from build123d import *

# Parameters (mm, degrees)
SKETCH1_R               = 8
BOSS_EXTRUDE1_DEPTH     = 26.25
SKETCH2_R               = 6
BOSS_EXTRUDE2_DEPTH     = 21.875
SKETCH3_R               = 6
BOSS_EXTRUDE3_DEPTH     = 21.875
CUT_EXTRUDE4_DEPTH      = 22.875
CUT_EXTRUDE4_DEPTH_BACK = 49.125
SKETCH7_W               = 1
SKETCH7_H               = 0.5
SKETCH9_R               = 3.175
CUT_EXTRUDE5_DEPTH      = 71
CHAMFER1_SIZE           = 1


with BuildPart() as part:
    # Sketch1 → Boss-Extrude1 (new body)
    with BuildSketch(Plane.XY):
        Circle(SKETCH1_R)
    extrude(amount=BOSS_EXTRUDE1_DEPTH)

    # Sketch2 → Boss-Extrude2 (add)
    with BuildSketch(Plane(origin=(0, 0, 0), x_dir=(-1, 0, 0), z_dir=(0, 0, -1))):
        Circle(SKETCH2_R)
    extrude(amount=BOSS_EXTRUDE2_DEPTH)

    # Sketch3 → Boss-Extrude3 (add)
    with BuildSketch(Plane.XY.offset(26.25)):
        Circle(SKETCH3_R)
    extrude(amount=BOSS_EXTRUDE3_DEPTH)

    # Sketch5 → Cut-Extrude4 (cut, two sides)
    with BuildSketch(Plane(origin=(0, 0, 0), x_dir=(-1, 0, 0), z_dir=(0, 0, -1))) as cut_extrude4_sk:
        with BuildLine():
            Line((-6, -5.291502622), (-6, 5.291502622))
            ThreePointArc((-6, 5.291502622), (-8, 0), (-6, -5.291502622))
        make_face()
        with BuildLine():
            ThreePointArc((8, 0), (7.483314774, 2.828427125), (6, 5.291502622))
            Line((6, 5.291502622), (6, -5.291502622))
            ThreePointArc((6, -5.291502622), (7.483314774, -2.828427125), (8, 0))
        make_face()
    extrude(amount=CUT_EXTRUDE4_DEPTH, mode=Mode.SUBTRACT)
    extrude(cut_extrude4_sk.sketch, amount=-CUT_EXTRUDE4_DEPTH_BACK, mode=Mode.SUBTRACT)

    # Sketch7 → Cut-Revolve1 (revolve, cut)
    with BuildSketch(Plane(origin=(0, 0, 0), x_dir=(0, 0, -1), z_dir=(1, 0, 0))):
        with Locations((20.375, 5.75)):
            Rectangle(SKETCH7_W, SKETCH7_H)
        with Locations((-46.625, 5.75)):
            Rectangle(SKETCH7_W, SKETCH7_H)
    revolve(axis=Axis((0, 0, 48.125), (0, 0, -1)), mode=Mode.SUBTRACT)

    # Sketch8 → Cut-Revolve2 (revolve, cut)
    with BuildSketch(Plane(origin=(0, 0, 0), x_dir=(0, 0, -1), z_dir=(1, 0, 0))):
        with BuildLine():
            Line((-24.25, 8), (-20.25, 8))
            ThreePointArc((-20.25, 8), (-22.25, 6), (-24.25, 8))
        make_face()
        with BuildLine():
            Line((-6, 8), (-2, 8))
            ThreePointArc((-2, 8), (-4, 6), (-6, 8))
        make_face()
    revolve(axis=Axis((0, 0, 48.125), (0, 0, -1)), mode=Mode.SUBTRACT)

    # Sketch9 → Cut-Extrude5 (cut, through all)
    with BuildSketch(Plane.XY.offset(48.125)):
        Circle(SKETCH9_R)
    extrude(amount=-CUT_EXTRUDE5_DEPTH, mode=Mode.SUBTRACT)

    # Chamfer1
    chamfer1_edges = [part.edges().sort_by_distance(p)[0] for p in [
        (-3.175, 0, -21.875),
        (-3.175, 0, 48.125),
    ]]
    chamfer(chamfer1_edges, length=CHAMFER1_SIZE)


solid = part.part
Geometry: final body of the model. Coordinates: model frame, mm. A direction names the side the tool comes from. Coordinates: 2 decimals unless noted, no trailing zeros. Loops run counter-clockwise (first coordinate to the right, second up) from the corner with the lowest first, then second, coordinate; pieces in that order, holes last. Notation, with made-up numbers: (68.25, 41) - (107.25, 41) arc R12 cw to (107.25, 45) - close; hole circle Ø3 at (54.5, 80). An arc over 180 degrees is marked (long way). Put each result on its own line as item: value. Start each with the question number.
Q1. Line query: line 1 (Z direction, x = -0.25, y = -7); line 2 (Y direction, x = 0, z = 1.5) (3 decimals); line 3 (Z direction, x = -3, y = 6). Output: solid intervals per line, ascending.
Q2. Pin query (flat end, axial travel): pin 1 Ø1.5 at (y, z) = (-1, -11.5) entering from -X; pin 2 Ø1.5 at (x, z) = (3.5, -12) entering from -Y; pin 3 Ø1 at (x, z) = (4, 23) entering from +Y. Return the tip coordinate at first contact, or that it passes through.
Q3. Set-up query: faces 1 (the flat face through (0.4, 6.4, 26.25)), 2 (the cylindrical face through (5.54, -2.3, 47.62)), 3 (the cylindrical face through (-5.54, -2.3, -21.37)), 4 (the flat face through (-5, -3, 46.125)). Return all of +Z, -Z, +X, -X, +Y, -Y with unobstructed straight access to the full face (end or side cutting, diameter ignored); none if empty.
Q4. Cut plane C-C, the plane z = -6.5. Return loops of the section in (x, y) (3 decimals).
Q5. Cut plane B-B, the plane y = 7. Give the number of separate pieces and of enclosed holes in the cut face, and give its area (3 significant figures).
Filled sheet:
1. line 1: 0 to 2.27, 5.73 to 20.52, 23.98 to 26.25
1. line 2: -8 to -3.175, 3.175 to 8
1. line 3: 0 to 2.47, 5.53 to 20.72, 23.78 to 26.25
2. pin 1: x = -5.99
2. pin 2: y = -5.33
2. pin 3: y = 5.18
3. face 1: +Z, +Y
3. face 2: +Z
3. face 3: -Z
3. face 4: none
4. outline: circle Ø12 at (0, 0); hole circle Ø6.35 at (0, 0)
5. separate pieces: 3
5. enclosed holes: 0
5. area: 146 mm²
